For this review, use the dimensioned drawing (mm, ordinates from the lowest corner) and the shaded views. Give positions to 0.01 mm unless a question says otherwise; leave off trailing zeros. Loops run counter-clockwise (first coordinate to the right, second up) from the corner with the lowest first, then second, coordinate; pieces in that order, holes last. Notation, with made-up numbers: M 34.5,-18 L 51.5,-18 A20 cw 51.5,12 Z; hole C -4,2 d2. An arc over 180 degrees is marked long. Use a Markdown table: item, result. Add a question column.
(1) Draft analysis for pull direction X (two halves, no side actions). For the marked faces 1, 2 and 3, state which applies: pulls with the +X half, pulls with the -X half, needs draft (parallel to the pull), parting line crosses it, or undercut.
(2) For probe 1 along X at (y, z) = (2.5, 0.3) (1 decimal); probe 2 along Y at (x, z) = (17.5, 1) (1 decimal); probe 3 along X at (y, z) = (16.5, 0.8) (1 decimal), list the stretches that pass through material, from the lowest coordinate up.
(3) Add section A-A, the plane y = 17.5. Give the boundary of the cut face in (x, z).
(4) Add section C-C, the plane z = 1.15. Give the boundary of the cut face in (x, y) (1 decimal).
(5) Add section D-D, the plane x = 28. Give the boundary of the cut face in (y, z), then the cut area to 3 significant figures.
(6) Add section B-B, the plane x = 14.5. Give the boundary of the cut face in (y, z).
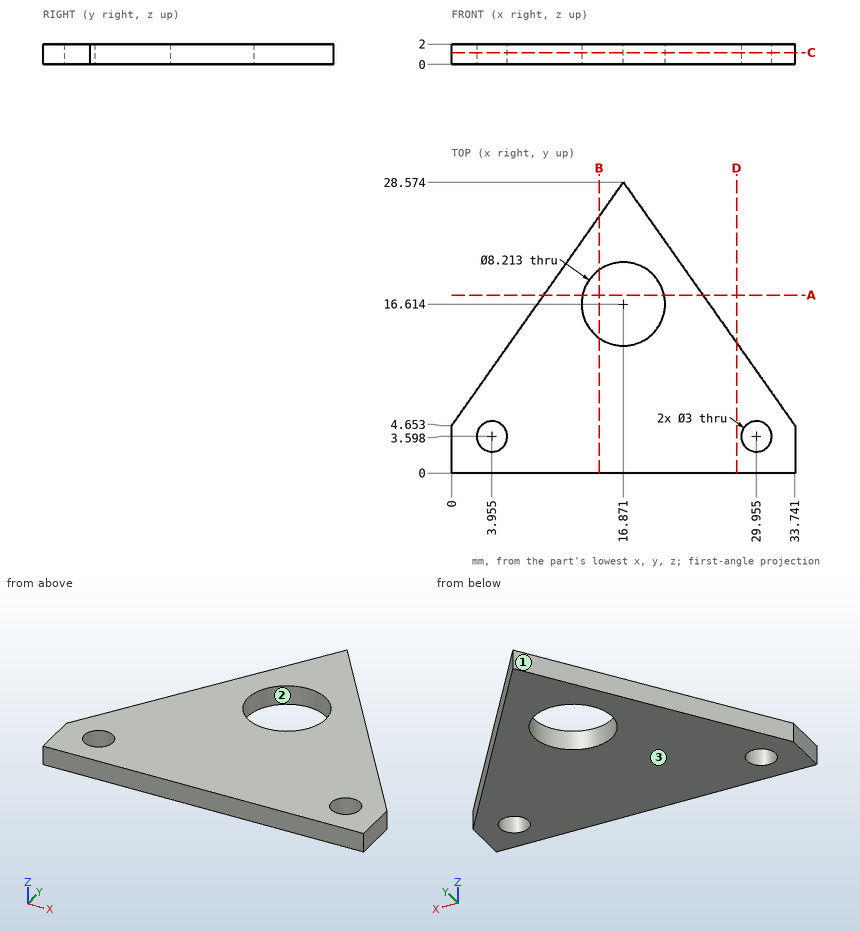
Established:
| question | item | result |
|---|---|---|
| 1 | face 1 | pulls with the -X half |
| 1 | face 2 | undercut |
| 1 | face 3 | needs draft |
| 2 | probe 1 | 0 to 2.9, 5 to 28.9, 31 to 33.7 |
| 2 | probe 2 | 0 to 12.6, 20.7 to 27.7 |
| 2 | probe 3 | 8.4 to 12.8, 21 to 25.4 |
| 3 | outline | M 9.06,0 L 12.86,0 L 12.86,2 L 9.06,2 Z; M 20.88,0 L 24.68,0 L 24.68,2 L 20.88,2 Z |
| 4 | outline | M 0,0 L 33.7,0 L 33.7,4.7 L 16.9,28.6 L 0,4.7 Z; hole C 4,3.6 d3; hole C 16.9,16.6 d8.2; hole C 30,3.6 d3 |
| 5 | outline | M 0,0 L 12.79,0 L 12.79,2 L 0,2 Z |
| 5 | area | 25.6 mm^2 |
| 6 | outline | M 0,0 L 13.26,0 L 13.26,2 L 0,2 Z; M 19.97,0 L 25.21,0 L 25.21,2 L 19.97,2 Z |
